Geometry: final body of the model. Coordinates: model frame, mm. A direction names the side the tool comes from. Coordinates: 2 decimals unless noted, no trailing zeros. Loops run counter-clockwise (first coordinate to the right, second up) from the corner with the lowest first, then second, coordinate; pieces in that order, holes last. Notation, with made-up numbers: (2.5, 23.5) -> (57.5, 23.5) arc R18 ccw to (57.5, 37.5) -> close; hole circle Ø8 at (68.5, 47.25). An arc over 180 degrees is marked (long way). One line per item, written item: value. Start each with the question number.
from build123d import *

# Parameters (mm, degrees)
F0_R     = 23.5
F0_R_2   = 15
F1_DEPTH = 10
F2_T     = -1
F3_R     = 1
F3_R_2   = 0.75
F4_DEPTH = 5
F5_R     = 0.75
F6_DEPTH = 1.1


with BuildPart() as f1:
    # F0 (on Top) → F1 (new body)
    with BuildSketch(Plane.XY):
        Circle(F0_R)
        Circle(F0_R_2, mode=Mode.SUBTRACT)
    extrude(amount=F1_DEPTH)

    # F2
    f2_openings = [f1.faces().sort_by_distance(p)[0] for p in [
        (-22.83532, 0, 10),
    ]]
    offset(amount=F2_T, openings=f2_openings)

    # F3 (on face) → F4 (join)
    with BuildSketch(Plane(origin=(0, 0, 0), x_dir=(1, 0, 0), z_dir=(0, 0, -1))):
        with Locations((-19.737165, -0.43914)):
            Circle(F3_R)
        with Locations((-19.737165, -0.43914)):
            Circle(F3_R_2, mode=Mode.SUBTRACT)
    extrude(amount=F4_DEPTH)

    # F5 (on face) → F6 (cut)
    with BuildSketch(Plane(origin=(0, 0, 0), x_dir=(1, 0, 0), z_dir=(0, 0, -1))):
        with Locations((-19.737165, -0.43914)):
            Circle(F5_R)
    extrude(amount=-F6_DEPTH, mode=Mode.SUBTRACT)


solid = f1.part
1. Pin query (flat end, axial travel): pin 1 Ø3 at (x, y) = (-3.5, 13.5) entering from -Z; pin 2 Ø6 at (x, z) = (-6.5, 4) entering from -Y; pin 3 Ø3 at (x, z) = (16.5, -2.5) entering from +Y; pin 4 Ø6 at (y, z) = (4, 4) entering from -X. Return the tip coordinate at first contact, or that it passes through.
2. Section C-C on z = 6.25. Return the cut outline in (x, y), plus the area to 3 significant figures.
3. Section A-A on x = 0. Return the cut outline in (y, z), plus the area to 3 significant figures.
4. Set-up query: faces 4 (the face through (-3.47, -15.62, 5.44)), 5 (the face through (-14.985, 0.66, 4.93)). Return all of +Z, -Z, +X, -X, +Y, -Y with unobstructed straight access to the full face (end or side cutting, diameter ignored); none if empty.
5. Section B-B on y = -2.5. Return the cut outline in (x, z), plus the area to 3 significant figures.
6. Line query: L1, parallel to Y at x = 0, z = 8.25; L2, parallel to X at y = -8.5, z = 3.75; L3, parallel to X at y = -9, z = 5.5. Output: solid intervals per line, ascending. Write a range as [from, to].
7. Draft query along Y for faces 1 (the face through (10.382, -19.961, 5.437)), 2 (the face through (-20.736, 0.395, -2.465)), 3 (the face through (0, -23, 10)). Return one class per face: released by +Y, released by -Y, zero draft, split by the parting line, or undercut.
8. Section D-D on y = -19.5. Return the cut outline in (x, z), plus the area to 3 significant figures.
Checks:
1. pin 1: z = 0
1. pin 2: y = -23.24
1. pin 3: through
1. pin 4: x = -23.48
2. outline: circle Ø47 at (0, 0); circle Ø32 at (0, 0); hole circle Ø45 at (0, 0); hole circle Ø30 at (0, 0)
2. area: 242 mm²
3. outline: (-23.5, 0) -> (-15, 0) -> (-15, 10) -> (-16, 10) -> (-16, 1) -> (-22.5, 1) -> (-22.5, 10) -> (-23.5, 10) -> close; (15, 0) -> (23.5, 0) -> (23.5, 10) -> (22.5, 10) -> (22.5, 1) -> (16, 1) -> (16, 10) -> (15, 10) -> close
3. area: 53.0 mm²
4. face 4: +Z
4. face 5: +Z, -Z
5. outline: (-23.37, 0) -> (-14.79, 0) -> (-14.79, 10) -> (-15.8, 10) -> (-15.8, 1) -> (-22.36, 1) -> (-22.36, 10) -> (-23.37, 10) -> close; (14.79, 0) -> (23.37, 0) -> (23.37, 10) -> (22.36, 10) -> (22.36, 1) -> (15.8, 1) -> (15.8, 10) -> (14.79, 10) -> close
5. area: 53.5 mm²
6. L1: [-23.5, -22.5], [-16, -15], [15, 16], [22.5, 23.5]
6. L2: [-21.91, -20.83], [-13.56, -12.36], [12.36, 13.56], [20.83, 21.91]
6. L3: [-21.71, -20.62], [-13.23, -12], [12, 13.23], [20.62, 21.71]
7. face 1: undercut
7. face 2: split by the parting line
7. face 3: zero draft
8. outline: (-13.11, 0) -> (13.11, 0) -> (13.11, 10) -> (11.22, 10) -> (11.22, 1) -> (-11.22, 1) -> (-11.22, 10) -> (-13.11, 10) -> close
8. area: 60.2 mm²
